```python
from build123d import *

# Parameters (mm, degrees)
SKETCH5_W            = 50
SKETCH5_H            = 25
SKETCH7_W            = 40
SKETCH7_H            = 21
SKETCH9_W            = 21
SKETCH9_H            = 40
BOSS_EXTRUDE2_DEPTH  = 560
SKETCH10_W           = 50
SKETCH10_H           = 25
BOSS_EXTRUDE3_DEPTH  = 560
SKETCH11_W           = 40
SKETCH11_H           = 25
BOSS_EXTRUDE4_DEPTH  = 590
BOSS_EXTRUDE7_REACH  = 1360.803
SKETCH13_W           = 21
SKETCH13_H           = 40
BOSS_EXTRUDE11_REACH = 1299.213
SKETCH19_R           = 12.5
SKETCH21_W           = 5
SKETCH21_H           = 25
BOSS_EXTRUDE13_DEPTH = 90
SKETCH22_R           = 5
CUT_EXTRUDE1_DEPTH   = 90


with BuildPart() as part:
    # Sweep3: sweep along a path in Sketch1
    with BuildLine(Plane.XY) as sweep3_path:
        Line((-345, 960), (345, 960))
        Line((345, 960), (345, -960))
        Line((345, -960), (-345, -960))
        Line((-345, -960), (-345, 960))
    # Sketch5 → Sweep3 (sweep)
    with BuildSketch(Plane(origin=(-345, 960, 0), x_dir=(0, 0, -1), z_dir=(1, 0, 0))):
        with Locations((25, -12.5)):
            Rectangle(SKETCH5_W, SKETCH5_H)
    sweep(path=sweep3_path.line, transition=Transition.RIGHT)

    # Sweep4: sweep along a path in Sketch6
    with BuildLine(Plane.XY) as sweep4_path:
        Line((-345, -260), (345, -260))
    # Sketch7 → Sweep4 (sweep)
    with BuildSketch(Plane(origin=(345, -260, 0), x_dir=(0, 0, -1), z_dir=(1, 0, 0))):
        with Locations((20, 10.5)):
            Rectangle(SKETCH7_W, SKETCH7_H)
    sweep(path=sweep4_path.line)

    # Sketch9 → Boss-Extrude2 (add)
    with BuildSketch(Plane.XY):
        with Locations((334.5, -249)):
            Rectangle(SKETCH9_W, SKETCH9_H)
    boss_extrude2 = extrude(amount=BOSS_EXTRUDE2_DEPTH)

    # Mirror1: Boss-Extrude2 across plane
    add(boss_extrude2.mirror(Plane(origin=(0, 0, 0), x_dir=(0, 0, 1), z_dir=(1, 0, 0))))

    # Sketch10 → Boss-Extrude3 (add)
    with BuildSketch(Plane.XY):
        with Locations((320, 947.5)):
            Rectangle(SKETCH10_W, SKETCH10_H)
    boss_extrude3 = extrude(amount=BOSS_EXTRUDE3_DEPTH)

    # Mirror3: Boss-Extrude3 across plane
    add(boss_extrude3.mirror(Plane(origin=(0, 0, 0), x_dir=(0, 0, 1), z_dir=(1, 0, 0))))

    # Sketch11 → Boss-Extrude4 (add)
    with BuildSketch(Plane(origin=(-295, 0, 0), x_dir=(0, 0, -1), z_dir=(1, 0, 0))):
        with Locations((-540, 947.5)):
            Rectangle(SKETCH11_W, SKETCH11_H)
    extrude(amount=BOSS_EXTRUDE4_DEPTH)

    # Sketch13 → Boss-Extrude7 (add, up to next)
    with BuildSketch(Plane(origin=(0, -229, 0), x_dir=(1, 0, 0), z_dir=(0, 1, 0)), mode=Mode.PRIVATE) as boss_extrude7_sk1:
        with Locations((-334.5, -440)):
            Rectangle(SKETCH13_W, SKETCH13_H)
    boss_extrude7_tool1 = extrude(boss_extrude7_sk1.sketch, amount=BOSS_EXTRUDE7_REACH, mode=Mode.PRIVATE) - part.part
    boss_extrude7 = boss_extrude7_tool1.solids().sort_by_distance((-334.5, -229, 440))[0]
    add(boss_extrude7)

    # Mirror7: Boss-Extrude7 across plane
    add(boss_extrude7.mirror(Plane(origin=(0, 0, 0), x_dir=(0, 0, 1), z_dir=(1, 0, 0))))

    # Sketch19 → Boss-Extrude11 (add, up to next)
    with BuildSketch(Plane(origin=(-324, 0, 0), x_dir=(0, 0, -1), z_dir=(1, 0, 0)), mode=Mode.PRIVATE) as boss_extrude11_sk1:
        with Locations(Location((-547.5, -249, 0), (0, 0, 180))):
            Circle(SKETCH19_R)
    boss_extrude11_tool1 = extrude(boss_extrude11_sk1.sketch, amount=BOSS_EXTRUDE11_REACH, mode=Mode.PRIVATE) - part.part
    add(boss_extrude11_tool1.solids().sort_by_distance((-324, -249, 547.5))[0])

    # Sketch21 → Boss-Extrude13 (add)
    with BuildSketch(Plane(origin=(0, 0, 520), x_dir=(-1, 0, 0), z_dir=(0, 0, -1))):
        with Locations((-7.5, 947.5)):
            Rectangle(SKETCH21_W, SKETCH21_H)
        with Locations((7.5, 947.5)):
            Rectangle(SKETCH21_W, SKETCH21_H)
    extrude(amount=BOSS_EXTRUDE13_DEPTH)

    # Sketch22 → Cut-Extrude1 (cut)
    with BuildSketch(Plane.ZY.offset(10)):
        with Locations(Location((440, 947.5, 0), (0, 0, 270))):
            Circle(SKETCH22_R)
    extrude(amount=-CUT_EXTRUDE1_DEPTH, mode=Mode.SUBTRACT)


solid = part.part
```
Source: CAD feature listing. Evaluate the final solid. Frame: model axes, mm. A direction names the side the tool comes from. Round coordinates to 2 decimals unless told otherwise and drop trailing zeros. Write each loop counter-clockwise with the first axis right and the second up, starting at its lowest first coordinate (ties: lowest second). Pieces come first, ordered by that corner, then holes. Notation, with made-up numbers: M -7,2 L 2,2 A22 cw 2,9 Z; hole C 51,54.5 d2. An arc over 180 degrees is marked long. Answer as a JSON object with one key per item and string values. Group by question number.
(1) Ray query, line 1 (Z direction, x = 8, y = 947); line 2 (Y direction, x = 6, z = 440). Return the intervals inside material, ascending. Write a range as [from, to].
(2) Section query A-A on x = -194.5. Output: boundary loops of the cut face in (y, z).
(3) Section query C-C on z = 24.5. Output: boundary loops of the cut face in (x, y), then the cut area to 3 significant figures.
(4) Section query D-D on y = -305.5. Output: boundary loops of the cut face in (x, z).
(5) Mould query, pull axis Y, two halves, no side actions, for faces 1 (the flat face through (-5, 960, 530)), 2 (the flat face through (4, -260, -20)), 3 (the flat face through (334, -4, -50)). Classes: +Y half, -Y half, draft (parallel to the pull), parting line (faces both ways), or undercut.
(6) Section query B-B on y = 166.5. Output: boundary loops of the cut face in (x, z), then the cut area to 3 significant figures.
(7) Reachability of faces 4 (the flat face through (4, -239, -20)), 5 (the flat face through (-4, -935, -25)), 6 (the flat face through (345, 138, -18)) from +Z, -Z, +X, -X, +Y, -Y: full face, straight path, thin tool, end or side. Return the list, or none.
Computed values:
{
 "1": {"line 1": "[-50, 0], [430, 435.03], [444.97, 560]", "line 2": "[935, 942.5], [952.5, 960]"},
 "2": {"outline": "M -960,-50 L -935,-50 L -935,0 L -960,0 Z; C -249,547.5 d25; M -260,-40 L -239,-40 L -239,0 L -260,0 Z; M 935,-50 L 960,-50 L 960,0 L 935,0 Z; M 935,520 L 960,520 L 960,560 L 935,560 Z"},
 "3": {"outline": "M -345,-269 L -324,-269 L -324,-229 L -345,-229 Z; M -345,935 L -295,935 L -295,960 L -345,960 Z; M 295,935 L 345,935 L 345,960 L 295,960 Z; M 324,-269 L 345,-269 L 345,-229 L 324,-229 Z", "area": "4,180 mm^2"},
 "4": {"outline": "M -345,-50 L -320,-50 L -320,0 L -345,0 Z; M 320,-50 L 345,-50 L 345,0 L 320,0 Z"},
 "5": {"face 1": "+Y half", "face 2": "undercut", "face 3": "draft"},
 "6": {"outline": "M -345,-50 L -320,-50 L -320,0 L -345,0 Z; M -345,420 L -324,420 L -324,460 L -345,460 Z; M 320,-50 L 345,-50 L 345,0 L 320,0 Z; M 324,420 L 345,420 L 345,460 L 324,460 Z", "area": "4,180 mm^2"},
 "7": {"face 4": "-Z", "face 5": "+Z, -Z", "face 6": "+Z, -Z, +X, +Y, -Y"}
}
